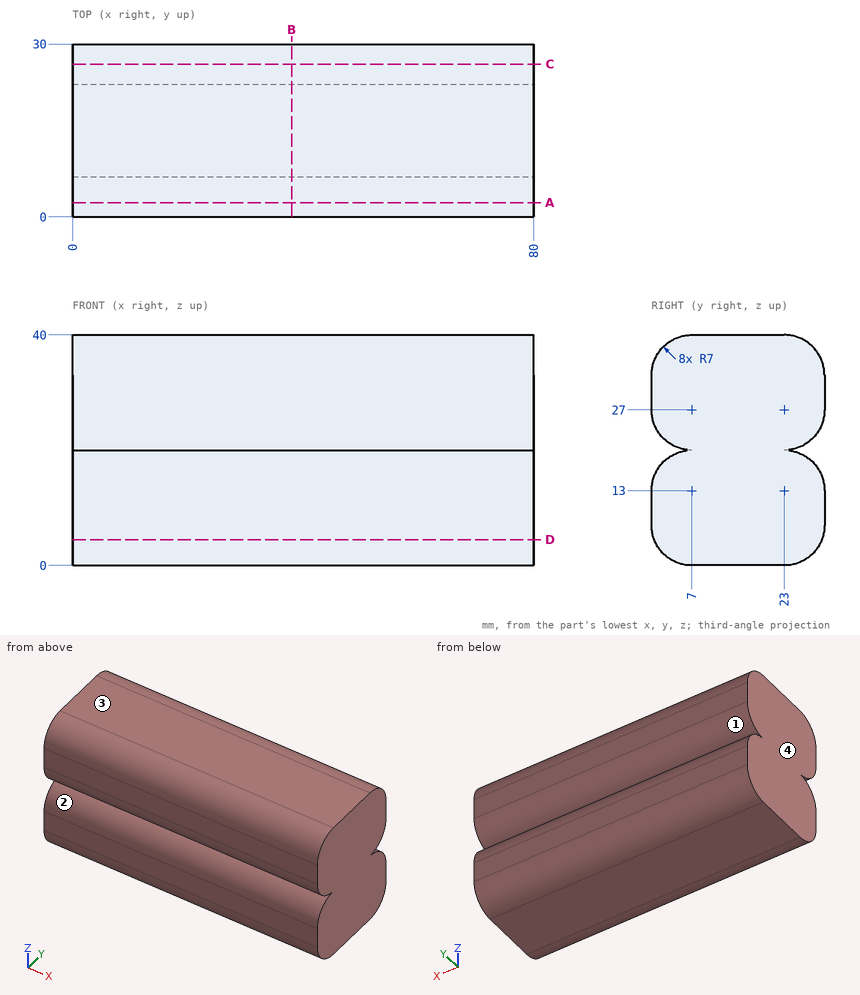
Part print with two shaded views. Sizes in mm from the minimum x, y, z corner. Coordinates: 2 decimals unless noted, no trailing zeros. Order: outer loops, then holes, each group sorted by start corner. A loop starts at its lowest first (then second) coordinate and runs counter-clockwise, first axis right, second up. Notation, with made-up numbers: M -16,-25 L 17,-25 A25 ccw 17,4 Z; hole C 51,-5.5 d3. An arc over 180 degrees is marked long. Use a Markdown table: item, result.
(1) Flat gauge pins, fed straight in: pin 1 (4 mm diameter, centred on x = 30.5, z = 17, fed in from +Y); pin 2 (3 mm diameter, centred on x = 67.5, z = 19.5, fed in from +Y); pin 3 (1.5 mm diameter, centred on x = 16.5, z = 17.5, fed in from -Y). Where does each tip first touch, or does it go through?
A:
| item | result |
|---|---|
| pin 1 | stops at y = 29.71 |
| pin 2 | stops at y = 27.9 |
| pin 3 | stops at y = 1.09 |
(2) Cut at B-B on x = 38. Write the cut outline in (y, z), then the cut area to 3 significant figures.
A:
| item | result |
|---|---|
| outline | M 0,7 A7 ccw 7,0 L 23,0 A7 ccw 30,7 L 30,13 A7 ccw 23,20 A7 ccw 30,27 L 30,33 A7 ccw 23,40 L 7,40 A7 ccw 0,33 L 0,27 A7 ccw 7,20 A7 ccw 0,13 Z |
| area | 1,120 mm^2 |
(3) Pull direction Z, two halves, no side cores. Call the marked faces 1, 2, 3 and 4: released by +Z, released by -Z, zero draft, split by the parting line, or undercut.
A:
| item | result |
|---|---|
| face 1 | undercut |
| face 2 | undercut |
| face 3 | released by +Z |
| face 4 | zero draft |
(4) Cut at A-A on y = 2.5. Write the cut outline in (x, z), then the cut area to 3 significant figures.
A:
| item | result |
|---|---|
| outline | M 0,1.64 L 80,1.64 L 80,18.36 L 0,18.36 Z; M 0,21.64 L 80,21.64 L 80,38.36 L 0,38.36 Z |
| area | 2,680 mm^2 |
(5) Probe L1, parallel to Y at x = 17, z = 13.5; L2, parallel to Z at x = 67, y = 28.75; L3, parallel to Z at x = 22, y = 2.5. List the from-to ranges inside material, lowest first.
A:
| item | result |
|---|---|
| L1 | y = 0.02 to 29.98 |
| L2 | z = 3.01 to 16.99, 23.01 to 36.99 |
| L3 | z = 1.64 to 18.36, 21.64 to 38.36 |
(6) Cut at C-C on y = 26.5. Write the cut outline in (x, z), then the cut area to 3 significant figures.
A:
| item | result |
|---|---|
| outline | M 0,0.94 L 80,0.94 L 80,19.06 L 0,19.06 Z; M 0,20.94 L 80,20.94 L 80,39.06 L 0,39.06 Z |
| area | 2,900 mm^2 |
(7) Cut at D-D on z = 4.5. Write the cut outline in (x, y), then the cut area to 3 significant figures.
A:
| item | result |
|---|---|
| outline | M 0,0.46 L 80,0.46 L 80,29.54 L 0,29.54 Z |
| area | 2,330 mm^2 |
